from build123d import *

# Parameters (mm, degrees)
PAD019_DEPTH = 12
FILLET005_R  = 2
FILLET006_R  = 2


with BuildPart() as part:
    # Sketch058 → Pad019 (new body)
    with BuildSketch(Plane.YZ):
        with BuildLine():
            Line((-110, 0), (-110, 20))
            Line((-110, 20), (-30, 70))
            Line((-30, 70), (30, 70))
            Line((30, 70), (110, 20))
            Line((110, 20), (110, 0))
            Line((110, 0), (80, 0))
            ThreePointArc((80, 0), (0, 56.277187), (-80, 0))
            Line((-110, 0), (-80, 0))
        make_face()
    extrude(amount=PAD019_DEPTH)

    # Fillet005
    fillet005_edges = [part.edges().sort_by_distance(p)[0] for p in [
        (0, 0, 56.277187),
        (12, 0, 56.277187),
    ]]
    fillet(fillet005_edges, radius=FILLET005_R)

    # Fillet006
    fillet006_edges = [part.edges().sort_by_distance(p)[0] for p in [
        (12, 70, 45),
        (0, 70, 45),
        (0, -70, 45),
        (12, -70, 45),
        (0, -110, 10),
        (12, -110, 10),
        (0, 110, 10),
        (12, 110, 10),
    ]]
    fillet(fillet006_edges, radius=FILLET006_R)


solid = part.part
Geometry check sheet. Reference: the model listing, model coordinates, mm. Round coordinates to 2 decimals unless told otherwise and drop trailing zeros. Write each loop counter-clockwise with the first axis right and the second up, starting at its lowest first coordinate (ties: lowest second). Pieces come first, ordered by that corner, then holes. Notation, with made-up numbers: (83, 32.25) - (137, 32.25) arc R25 ccw to (137, 60.25) - close; hole circle Ø2 at (79, 77). An arc over 180 degrees is marked (long way). One line per item, written item: value.
1. Mould release check, pull along Y, two halves, no side actions. Record for faces 1 (the face through (5.944, 1.459, 56.265)), 2 (the face through (6, -110, 10)), 3 (the face through (12, 0.5, 58.5)): released by +Y, released by -Y, zero draft, split by the parting line, or undercut.
The answers:
face 1: undercut
face 2: released by -Y
face 3: zero draft
2. Cross-section at A-A on x = 6.25. Record the boundary of the cut face in (y, z), and give its area (3 significant figures).
The answers:
outline: (-110, 0) - (-80, 0) arc R85 cw to (80, 0) - (110, 0) - (110, 20) - (30, 70) - (-30, 70) - (-110, 20) - close
area: 4,840 mm^2
3. Scan lines: L1, parallel to Y at x = 7, z = 46.5; L2, parallel to Y at x = 2.5, z = 47; L3, parallel to Z at x = 9.5, y = -78.5. Record each from-to range of solid material in increasing order.
The answers:
L1: y = -67.6 to -39.58, 39.58 to 67.6
L2: y = -66.8 to -38.61, 38.61 to 66.8
L3: z = 3.88 to 39.69
4. Depth check by flat-ended pin: pin 1 Ø3 at (x, z) = (5, 46) entering from +Y; pin 2 Ø1.5 at (x, z) = (6, 55.5) entering from -Y; pin 3 Ø2 at (x, z) = (2.5, 39) entering from +Y. Enter the tip coordinate at first touch or a pass-through.
The answers:
pin 1: stops at y = 70.8
pin 2: stops at y = -54.4
pin 3: stops at y = 81.2
